Autodesk Inventor part; units mm, degrees
ref_plane "Plano de trabalho1" through (0, 4.5, 0) normal (0, 1, 0) x (-1, 0, 0)
ref_plane "YZ Plane" through (0, 0, 0) normal (1, 0, 0) x (0, 1, 0)
ref_plane "XY Plane" through (0, 0, 0) normal (0, 0, 1) x (1, 0, 0)
sketch "Esboço1" plane through (0, 0, 0) normal (0, 0, 1) x (1, 0, 0)
  circle A0 centre (0, 0) radius 4.5
  dimension "d0" = 9
extrude "Extrusão1" add sketch "Esboço1" along normal mid plane 38
sketch "Esboço2" plane through (0, 0, 19) normal (0, 0, 1) x (1, 0, 0)
  point P0 (0, 0)
  point P1 (0, 0)
hole "Furo1" at (0, 0, 19) direction (0, 0, -1) diameter 3.2 depth 7 tip angle 118
sketch "Esboço3" plane through (0, 0, -19) normal (0, 0, -1) x (-1, 0, 0)
  point P0 (0, 0)
  point P1 (0, 0)
hole "Furo2" at (0, 0, -19) direction (0, 0, 1) diameter 6.5 depth 27 tip angle 118
sketch "Esboço4" plane through (0, 0, -19) normal (0, 0, -1) x (-1, 0, 0)
  circle A0 centre (0, 0) radius 4.5
  circle A1 centre (0, 0) radius 4
  dimension "d18" = 8
extrude "Extrusão2" cut sketch "Esboço4" against normal blind 12
sketch "Esboço5" plane through (0, 0, 0) normal (1, 0, 0) x (0, 1, 0)
  line L0 (4.5, -7) -> (4.5, 19)
  line L1 (4.5, 1) -> (-4.5, 1)
  line L2 (-4.5, 1) -> (-4.5, -19)
  line L3 (4.5, -19) -> (4.5, 1)
  line L4 (-4.5, -7) -> (-4.5, 19)
  line L5 (-4, -19) -> (4, -19)
  line L6 (4, -19) -> (4, -7)
  line L7 (4.5, -19) -> (-4.5, -19)
  point P0 (0, 0)
  dimension "d23" = 20
extrude "Extrusão3" cut sketch "Esboço5" along normal mid plane 0.5
sketch "Esboço6" plane through (0, 0, 0) normal (0, 1, 0) x (-1, 0, 0)
  line L0 (-4.5, -7) -> (-4.5, 19)
  line L1 (4.5, -7) -> (4.5, 19)
  line L2 (-0.25, 1) -> (0.25, 1)
  line L3 (-4.5, -19) -> (4.5, -19)
  line L4 (4.5, -19) -> (4.5, 1)
  line L5 (4.5, 1) -> (-4.5, 1)
  line L6 (-4.5, 1) -> (-4.5, -19)
  line L7 (-4, -19) -> (-0.25, -19)
  line L8 (0.25, -19) -> (4, -19)
  line L9 (0.25, 1) -> (-0.25, 1)
  point P0 (0, 0)
extrude "Extrusão4" cut sketch "Esboço6" along normal mid plane 0.5
ref_plane "Plano de trabalho1" through (0, 4.5, 0) normal (0, 1, 0) x (-1, 0, 0)
sketch "Esboço7" plane through (0, 4.5, 0) normal (0, 1, 0) x (-1, 0, 0)
  line L0 (-1.6, 19) -> (1.6, 19)
  line L1 (0, 19) -> (0, 16) construction
  point P0 (0, 0)
  dimension "d28" = 3
hole "Furo3" at (0, 4.5, 16) direction (0, -1, 0) diameter 2.459 end up to surface
chamfer "Chanfro1" distance 0.5 angle 45 5 edges at (-4.5, 0, 19) (-2.8284, 2.8284, -19) (-2.8284, -2.8284, -19) (2.8284, -2.8284, -19) (2.8284, 2.8284, -19)
properties part number "N4049_pino_contato_T"
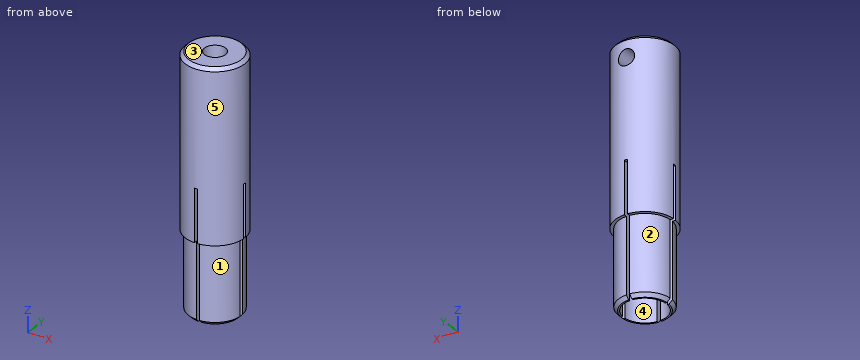
Verification items for the finished model (mm, model axes). Face numbers are marked on the shaded views. A direction names the side the tool comes from. Give positions to 0.01 mm unless a question says otherwise; leave off trailing zeros. Order: outer loops, then holes, each group sorted by start corner. A loop starts at its lowest first (then second) coordinate and runs counter-clockwise, first axis right, second up. Notation, with made-up numbers: (60.25, 70.5) - (101.25, 70.5) arc R26 cw to (101.25, 101.5) - close; hole circle Ø6 at (-0.5, 47). An arc over 180 degrees is marked (long way). Answer as CSV lines item,"result". Start each with the question number.
Item 1: Section check A-A, the plane z = -1.5. Record the boundary of the cut face in (x, y).
Item 2: Gauge pin test, flat ends, axial feed: pin 1 (1.5 mm diameter, centred on x = 3, z = -3.5, fed in from +Y); pin 2 (1 mm diameter, centred on y = -4, z = -4.5, fed in from +X); pin 3 (2 mm diameter, centred on x = 0, z = 16, fed in from +Y). Record the tip position at first contact, or that the pin passes through.
Item 3: Section check B-B, the plane z = -13. Record the boundary of the cut face in (x, y), plus the area to 3 significant figures.
Item 4: Section check C-C, the plane z = 16.5. Record the boundary of the cut face in (x, y).
Item 5: Access from +Z, -Z, +X, -X, +Y, -Y to the whole of each face (thin tool, end or side, straight path). Record for the marked faces 1, 2, 3, 4 and 5.
Item 6: Material ranges on L1, parallel to Y at x = -0.25, z = 6; L2, parallel to X at y = 3.1, z = 16, recorded low to high.
Filled in:
1,outline,"(-4.49, -0.25) arc R4.5 ccw to (-0.25, -4.49) - (-0.25, -3.24) arc R3.25 cw to (-3.24, -0.25) - close; (-4.49, 0.25) - (-3.24, 0.25) arc R3.25 cw to (-0.25, 3.24) - (-0.25, 4.49) arc R4.5 ccw to start; (0.25, -4.49) arc R4.5 ccw to (4.49, -0.25) - (3.24, -0.25) arc R3.25 cw to (0.25, -3.24) - close; (0.25, 3.24) arc R3.25 cw to (3.24, 0.25) - (4.49, 0.25) arc R4.5 ccw to (0.25, 4.49) - close"
2,pin 1,"y = 3.9"
2,pin 2,"x = 2.83"
2,pin 3,"y = -1.25"
3,outline,"(-3.99, -0.25) arc R4 ccw to (-0.25, -3.99) - (-0.25, -3.24) arc R3.25 cw to (-3.24, -0.25) - close; (-3.99, 0.25) - (-3.24, 0.25) arc R3.25 cw to (-0.25, 3.24) - (-0.25, 3.99) arc R4 ccw to start; (0.25, -3.99) arc R4 ccw to (3.99, -0.25) - (3.24, -0.25) arc R3.25 cw to (0.25, -3.24) - close; (0.25, 3.24) arc R3.25 cw to (3.24, 0.25) - (3.99, 0.25) arc R4 ccw to (0.25, 3.99) - close"
3,area,"15.6 mm^2"
4,outline,"(-1.12, 1.14) - (-1.12, 4.36) arc R4.5 ccw (long way) to (1.12, 4.36) - (1.12, 1.14) arc R1.6 cw (long way) to start"
5,face 1,"-Z, +X, -Y"
5,face 2,"-Z, -X, +Y"
5,face 3,"+Z, +X, -X, +Y, -Y"
5,face 4,"-Z"
5,face 5,"+Z, -Z"
6,L1,"-4.49 to -3.24, 3.24 to 4.49"
6,L2,"-3.26 to -1.23, 1.23 to 3.26"
